The figure shows three views and two pictorial views of one solid part (mm, origin at its lowest corner). Answer the questions. A direction names the side the tool comes from. Round coordinates to 2 decimals unless told otherwise and drop trailing zeros. Write each loop counter-clockwise with the first axis right and the second up, starting at its lowest first coordinate (ties: lowest second). Pieces come first, ordered by that corner, then holes. Notation, with made-up numbers: M 45,-19 L 81,-19 A24 cw 81,5 Z; hole C -1,8.25 d7. An arc over 180 degrees is marked long. Answer in a Markdown table with one row per item.
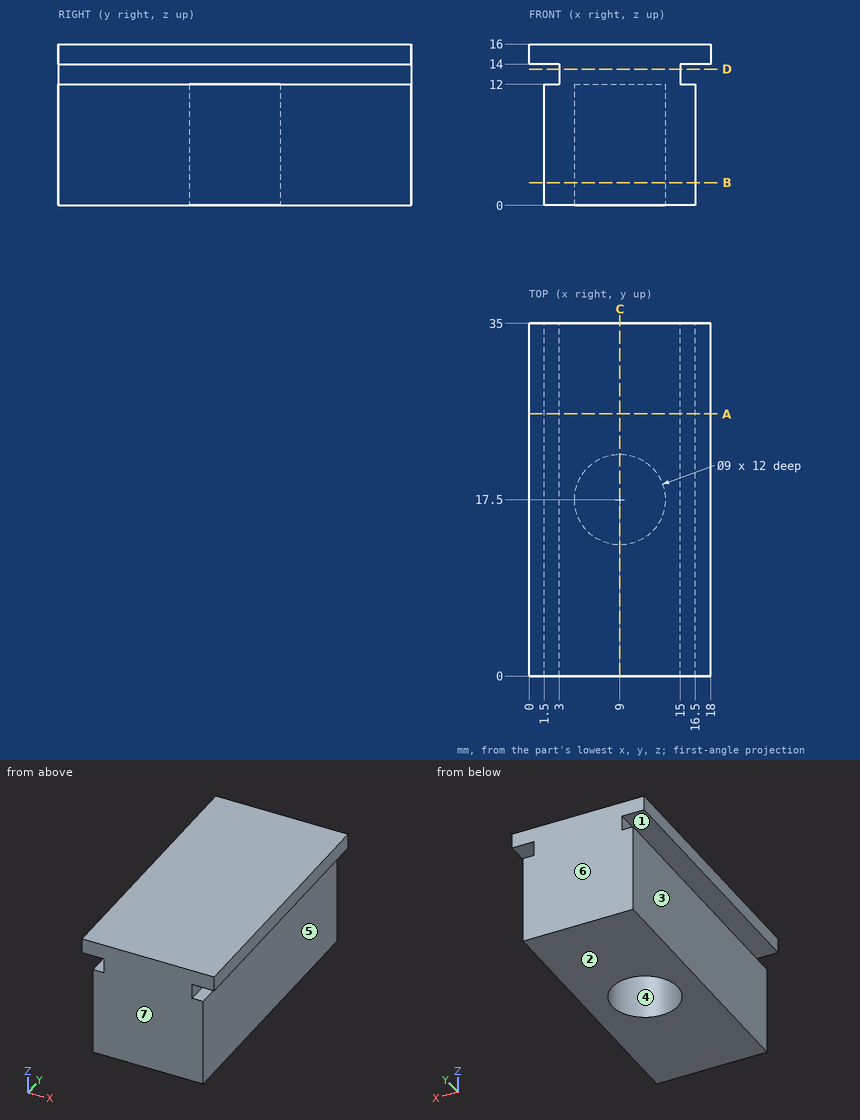
1. Determine the mould class of the marked faces 4, 5, 6 and 7 for opening direction Y: released by +Y, released by -Y, zero draft, split by the parting line, or undercut.
Calculated:
| item | result |
|---|---|
| face 4 | undercut |
| face 5 | zero draft |
| face 6 | released by +Y |
| face 7 | released by -Y |
2. Consider line 1 along Z through (x, y) = (2.75, 29.5); line 2 along Y through (x, z) = (9, 9.75); line 3 along Z through (x, y) = (9.25, 14.5). Determine where each line is inside the solid, lowest interval first. Write a range as from..to.
Calculated:
| item | result |
|---|---|
| line 1 | z = 0..12, 14..16 |
| line 2 | y = 0..13, 22..35 |
| line 3 | z = 12..16 |
3. A tool of negligible diameter and unlimited length cuts with its end or side. For the marked faces 1, 2 and 3, from which of +Z, -Z, +X, -X, +Y, -Y can it reach the whole face along a straight path? Write none if from no direction.
Calculated:
| item | result |
|---|---|
| face 1 | -X, +Y, -Y |
| face 2 | -Z, +X, -X, +Y, -Y |
| face 3 | -Z, -X, +Y, -Y |
4. The part is cut by section A-A (y = 26). Determine the outline of the cut face in (x, z), plus the area to 3 significant figures.
Calculated:
| item | result |
|---|---|
| outline | M 0,14 L 3,14 L 3,12 L 1.5,12 L 1.5,0 L 16.5,0 L 16.5,12 L 15,12 L 15,14 L 18,14 L 18,16 L 0,16 Z |
| area | 240 mm² |
5. The part is cut by section D-D (z = 13.5). Determine the outline of the cut face in (x, y), plus the area to 3 significant figures.
Calculated:
| item | result |
|---|---|
| outline | M 3,0 L 15,0 L 15,35 L 3,35 Z |
| area | 420 mm² |
6. Given pin 1 (6 mm diameter, centred on y = 13, z = 9, fed in from +X); pin 2 (9.5 mm diameter, centred on y = 11.5, z = 4, fed in from -X), each flat-ended and moving along its own axis, determine where each tip first touches the part or whether it passes through.
Calculated:
| item | result |
|---|---|
| pin 1 | stops at x = 16.5 |
| pin 2 | stops at x = 1.5 |
7. The part is cut by section C-C (x = 9). Determine the outline of the cut face in (y, z), plus the area to 3 significant figures.
Calculated:
| item | result |
|---|---|
| outline | M 0,0 L 13,0 L 13,12 L 22,12 L 22,0 L 35,0 L 35,16 L 0,16 Z |
| area | 452 mm² |
8. The part is cut by section B-B (z = 2.25). Determine the outline of the cut face in (x, y), plus the area to 3 significant figures.
Calculated:
| item | result |
|---|---|
| outline | M 1.5,0 L 16.5,0 L 16.5,35 L 1.5,35 Z; hole C 9,17.5 d9 |
| area | 461 mm² |
